Input: dimensioned drawing with shaded views. Units: mm. Origin: part minimum x, y, z. Coordinates: 2 decimals unless noted, no trailing zeros. Loops run counter-clockwise (first coordinate to the right, second up) from the corner with the lowest first, then second, coordinate; pieces in that order, holes last. Notation, with made-up numbers: (41.5, 86.5) - (76.5, 86.5) arc R18 ccw to (76.5, 101.5) - close; hole circle Ø11 at (26, 26). An arc over 180 degrees is marked (long way). Put each result on its own line as item: value. Start each with the question number.
1) Section B-B on x = 20. Output: boundary loops of the cut face in (y, z).
2) Section D-D on x = 47.5. Output: boundary loops of the cut face in (y, z) (1 decimal).
3) Draft query along Y for the marked faces 1, 2 and 3. Return one class per face: +Y half, -Y half, draft (parallel to the pull), parting line (faces both ways), or undercut.
4) Material intervals for line 1 along Y through (x, z) = (4.72, 50.9); line 2 along Y through (x, z) = (69, 51) (1 decimal); line 3 along Z through (x, y) = (55, 28.5), sorted ascending. Write a range as from..to.
5) Contact query for flat-ended pins moving along their axis: pin 1 Ø2 at (x, y) = (4.72, 4.66) entering from -Z; pin 2 Ø1.5 at (x, z) = (38.5, 5.5) entering from -Y (1 decimal); pin 3 Ø4 at (x, y) = (45, 28.5) entering from -Z. Output: stop coordinate, or through.
6) Section A-A on x = 69.72. Output: boundary loops of the cut face in (y, z).
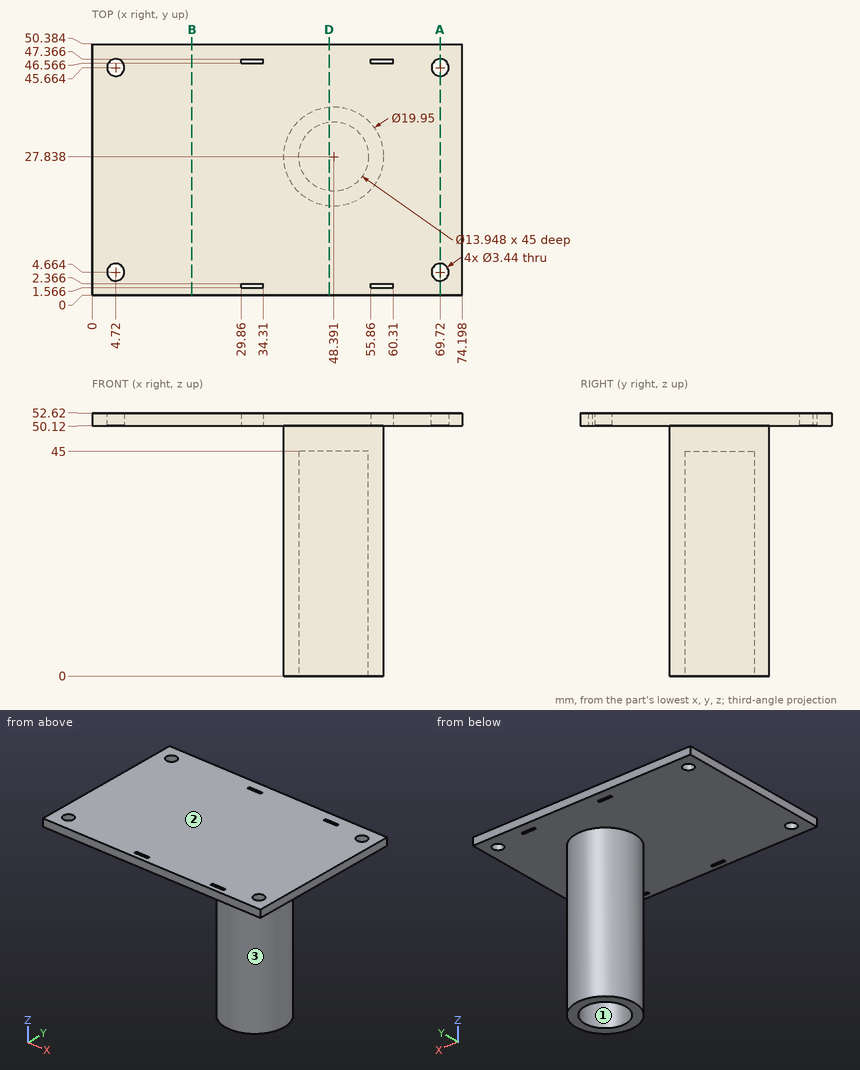
Answer block:
1. outline: (0, 50.12) - (50.38, 50.12) - (50.38, 52.62) - (0, 52.62) - close
2. outline: (0, 50.1) - (17.9, 50.1) - (17.9, 0) - (20.9, 0) - (20.9, 45) - (34.8, 45) - (34.8, 0) - (37.8, 0) - (37.8, 50.1) - (50.4, 50.1) - (50.4, 52.6) - (0, 52.6) - close
3. face 1: undercut
3. face 2: draft
3. face 3: parting line
4. line 1: y = 0..2.94, 6.38..43.94, 47.38..50.38
4. line 2: y = 0..3.1, 6.2..44.1, 47.2..50.4
4. line 3: z = 45..52.62
5. pin 1: passes through
5. pin 2: stops at y = 23.8
5. pin 3: stops at z = 45
6. outline: (0, 50.12) - (2.94, 50.12) - (2.94, 52.62) - (0, 52.62) - close; (6.38, 50.12) - (43.94, 50.12) - (43.94, 52.62) - (6.38, 52.62) - close; (47.38, 50.12) - (50.38, 50.12) - (50.38, 52.62) - (47.38, 52.62) - close
